```python
from build123d import *

# Parameters (mm, degrees)
SKETCH_2_W                       = 970
SKETCH_2_H                       = 100
SM_BASE_FLANGE_1_DEPTH           = 2
SM_EDGE_FLANGE_1_STRIP_W         = 44
SM_EDGE_FLANGE_1_STRIP_H         = 2
SM_EDGE_FLANGE_1_STRIP_CUT_DEPTH = 970
SM_EDGE_FLANGE_1_DEPTH           = 970
SM_EDGE_FLANGE_2_STRIP_W         = 9.4732
SM_EDGE_FLANGE_2_STRIP_H         = 2
SM_EDGE_FLANGE_2_STRIP_CUT_DEPTH = 970
SM_EDGE_FLANGE_2_DEPTH           = 970
SM_EDGE_FLANGE_3_STRIP_W         = 9.4732
SM_EDGE_FLANGE_3_STRIP_H         = 2
SM_EDGE_FLANGE_3_STRIP_CUT_DEPTH = 970
SM_EDGE_FLANGE_3_DEPTH           = 970
SKETCH_16_R                      = 7.5
CUT_EXTRUDE_1_DEPTH              = 10
SKETCH_17_R                      = 7.5
CUT_EXTRUDE_2_DEPTH              = 10


# Sheet-metal steps are written as plain solids
with BuildPart() as part:
    # Sketch 2 → 基体-法兰1 (new body)
    with BuildSketch(Plane.XY):
        Rectangle(SKETCH_2_W, SKETCH_2_H)
    extrude(amount=-SM_BASE_FLANGE_1_DEPTH)

    # 边线-法兰1 strip (across the edge) → 边线-法兰1 strip cut (cut)
    with BuildSketch(Plane(origin=(-485, -50, 0), x_dir=(0, 1, 0), z_dir=(1, 0, 0))):
        with Locations((-2, -1)):
            Rectangle(SM_EDGE_FLANGE_1_STRIP_W, SM_EDGE_FLANGE_1_STRIP_H)
    extrude(amount=SM_EDGE_FLANGE_1_STRIP_CUT_DEPTH, mode=Mode.SUBTRACT)

    # 边线-法兰1 section (across the edge) → 边线-法兰1 (add)
    with BuildSketch(Plane(origin=(-485, -50, 0), x_dir=(0, 1, 0), z_dir=(1, 0, 0))):
        with BuildLine():
            Line((0, 18), (0, 98))
            Line((0, 98), (2, 98))
            Line((2, 98), (2, 18))
            ThreePointArc((2, 18), (7.272077939, 5.272077939), (20, 0))
            Line((20, 0), (20, -2))
            ThreePointArc((20, -2), (5.857864376, 3.857864376), (0, 18))
        make_face()
    extrude(amount=SM_EDGE_FLANGE_1_DEPTH)

    # 边线-法兰2 strip (across the edge) → 边线-法兰2 strip cut (cut)
    with BuildSketch(Plane(origin=(485, 50, 0), x_dir=(0, -1, 0), z_dir=(-1, 0, 0))):
        with Locations((-2, -1)):
            Rectangle(SM_EDGE_FLANGE_2_STRIP_W, SM_EDGE_FLANGE_2_STRIP_H)
    extrude(amount=SM_EDGE_FLANGE_2_STRIP_CUT_DEPTH, mode=Mode.SUBTRACT)

    # 边线-法兰2 section (across the edge) → 边线-法兰2 (add)
    with BuildSketch(Plane(origin=(485, 50, 0), x_dir=(0, -1, 0), z_dir=(-1, 0, 0))):
        with BuildLine():
            Line((0, 0.7366), (0, 28))
            Line((0, 28), (2, 28))
            Line((2, 28), (2, 0.7366))
            ThreePointArc((2, 0.7366), (2.215745145, 0.215745145), (2.7366, 0))
            Line((2.7366, 0), (2.7366, -2))
            ThreePointArc((2.7366, -2), (0.801531583, -1.198468417), (0, 0.7366))
        make_face()
    extrude(amount=SM_EDGE_FLANGE_2_DEPTH)

    # 边线-法兰3 strip (across the edge) → 边线-法兰3 strip cut (cut)
    with BuildSketch(Plane(origin=(-485, -48, 98), x_dir=(0, 0, -1), z_dir=(1, 0, 0))):
        with Locations((-2, -1)):
            Rectangle(SM_EDGE_FLANGE_3_STRIP_W, SM_EDGE_FLANGE_3_STRIP_H)
    extrude(amount=SM_EDGE_FLANGE_3_STRIP_CUT_DEPTH, mode=Mode.SUBTRACT)

    # 边线-法兰3 section (across the edge) → 边线-法兰3 (add)
    with BuildSketch(Plane(origin=(-485, -48, 98), x_dir=(0, 0, -1), z_dir=(1, 0, 0))):
        with BuildLine():
            Line((0, 0.7366), (0, 28))
            Line((0, 28), (2, 28))
            Line((2, 28), (2, 0.7366))
            ThreePointArc((2, 0.7366), (2.215745145, 0.215745145), (2.7366, 0))
            Line((2.7366, 0), (2.7366, -2))
            ThreePointArc((2.7366, -2), (0.801531583, -1.198468417), (0, 0.7366))
        make_face()
    extrude(amount=SM_EDGE_FLANGE_3_DEPTH)

    # 草图16 → 切除-拉伸1 (cut)
    with BuildSketch(Plane(origin=(0, 50, 0), x_dir=(1, 0, 0), z_dir=(0, 1, 0))):
        with Locations(Location((-455, -15, 0), (0, 0, 270))):
            Circle(SKETCH_16_R)
    extrude(amount=-CUT_EXTRUDE_1_DEPTH, mode=Mode.SUBTRACT)

    # 草图17 → 切除-拉伸2 (cut)
    with BuildSketch(Plane.XY.offset(98)):
        with Locations((-455, -33)):
            Circle(SKETCH_17_R)
    extrude(amount=-CUT_EXTRUDE_2_DEPTH, mode=Mode.SUBTRACT)


solid = part.part
```
Source: CAD feature listing. Evaluate the final solid. Frame: model axes, mm. A direction names the side the tool comes from. Give positions to 0.01 mm unless a question says otherwise; leave off trailing zeros. Write each loop counter-clockwise with the first axis right and the second up, starting at its lowest first coordinate (ties: lowest second). Pieces come first, ordered by that corner, then holes.
1. Section query C-C (z = 62). Return the cut outline in (x, y), then the cut area to 3 significant figures.
2. Material intervals for line 1 along Y through (x, z) = (368.5, 18.5); line 2 along X through (y, z) = (49.05, 15); line 3 along Z through (x, y) = (-197, -30), sorted ascending.
3. First-contact query: pin 1 (10 mm diameter, centred on x = 14.5, z = 37.5, fed in from +Y); pin 2 (23 mm diameter, centred on x = 155, y = 6.5, fed in from +Z); pin 3 (1 mm diameter, centred on x = -20, z = 97, fed in from +Y). Flat tips, straight axial feed; report the tip coordinate or a pass-through.
4. Pull-direction query (Z, two-part tool) for faces 4 (the face through (485, 7.6, -0.4)), 5 (the face through (-6.79, -43.986, 3.703)), 6 (the face through (-462.32, 49.01, 13.37)), 7 (the face through (-7, -48, 57)); classes: +Z half, -Z half, draft (parallel to the pull), parting line (faces both ways), or undercut.
5. Section query B-B (y = 31.5). Return the cut outline in (x, z), then the cut area to 3 significant figures.
6. Section query A-A (x = -264.5). Return the cut outline in (y, z), then the cut area to 3 significant figures.
7. Access query for faces 1 (the face through (-448.07, -35.87, 97.01)), 2 (the face through (-6.79, -42.867, 5.413)), 3 (the face through (7, 48, 15)). Directions: +Z, -Z, +X, -X, +Y, -Y. A direction counts if a zero-diameter tool reaches every point of the face in a straight line with its end or side. Return the directions, or none.
Output values:
1. outline: (-485, -50) - (485, -50) - (485, -48) - (-485, -48) - close
1. area: 1,940 mm2
2. line 1: y = -50 to -48, 48 to 50
2. line 2: x = -485 to -462.5, -447.5 to 485
2. line 3: z = -2 to 0, 96 to 98
3. pin 1: stops at y = -48
3. pin 2: stops at z = 0
3. pin 3: stops at y = -20
4. face 4: draft
4. face 5: -Z half
4. face 6: undercut
4. face 7: undercut
5. outline: (-485, -2) - (485, -2) - (485, 0) - (-485, 0) - close
5. area: 1,940 mm2
6. outline: (-50, 18) arc R20 ccw to (-30, -2) - (47.26, -2) arc R2.74 ccw to (50, 0.74) - (50, 28) - (48, 28) - (48, 0.74) arc R0.74 cw to (47.26, 0) - (-30, 0) arc R18 cw to (-48, 18) - (-48, 95.26) arc R0.74 cw to (-47.26, 96) - (-20, 96) - (-20, 98) - (-47.26, 98) arc R2.74 ccw to (-50, 95.26) - close
6. area: 489 mm2
7. face 1: +Z
7. face 2: +X, -X
7. face 3: +Z, +X, -X
